Geometry: final body of the model. Coordinates: model frame, mm. Face numbers are marked on the shaded views. A direction names the side the tool comes from. Give positions to 0.01 mm unless a question says otherwise; leave off trailing zeros. Write each loop counter-clockwise with the first axis right and the second up, starting at its lowest first coordinate (ties: lowest second). Pieces come first, ordered by that corner, then holes. Notation, with made-up numbers: M 72.5,85.5 L 83.5,85.5 A15 ccw 83.5,104.5 Z; hole C 74,83.5 d1. An arc over 180 degrees is marked long. One line per question, with ' | ' between items.
Autodesk Inventor part; units mm, degrees
ref_plane "YZ Plane" through (0, 0, 0) normal (1, 0, 0) x (0, 1, 0)
ref_plane "XZ Plane" through (0, 0, 0) normal (0, 1, 0) x (-1, 0, 0)
ref_plane "XY Plane" through (0, 0, 0) normal (0, 0, 1) x (1, 0, 0)
sketch "Sketch1" plane through (0, 0, 0) normal (0, 1, 0) x (-1, 0, 0)
  line L0 (0, 0) -> (25.4, 0)
  line L1 (25.4, 0) -> (25.4, -50.8)
  line L2 (25.4, -50.8) -> (0, -50.8)
  line L3 (0, -50.8) -> (0, 0)
  dimension "d0" = 25.4
  dimension "d1" = 50.8
extrude "Extrusion1" add sketch "Sketch1" along normal blind 15.24
shell "Shell1" thickness 2.54 removed faces 1 at (-8.4667, 15.24, -33.8667)
sketch "Sketch3" plane through (-25.4, 0, 0) normal (0, 0, 1) x (1, 0, 0)
  line L0 (19.05, 4.064) -> (6.35, 4.064)
  line L1 (6.35, 4.064) -> (6.35, 9.144)
  line L2 (6.35, 9.144) -> (19.05, 9.144)
  line L3 (19.05, 9.144) -> (19.05, 4.064)
  point P0 (25.4, 0)
  dimension "d20" = 4.064
  dimension "d21" = 12.7
  dimension "d22" = 5.08
  dimension "d23" = 6.35
extrude "Extrusion3" cut sketch "Sketch3" against normal blind 2.54
chamfer "Chamfer1" distance 3.175 angle 45 2 edges at (-19.05, 9.144, -1.27) (-6.35, 9.144, -1.27)
sketch "Sketch5" plane through (-22.86, 2.54, -2.54) normal (0, 1, 0) x (1, 0, 0)
  line L0 (0, 0) -> (5.08, 0)
  line L1 (5.08, 0) -> (5.08, 45.72)
  line L2 (5.08, 45.72) -> (0, 45.72)
  line L3 (0, 45.72) -> (0, 0)
  line L4 (0, 45.72) -> (20.32, 45.72)
  line L5 (20.32, 0) -> (15.24, 0)
  line L6 (15.24, 0) -> (15.24, 45.72)
  line L7 (15.24, 45.72) -> (20.32, 45.72)
  line L8 (20.32, 45.72) -> (20.32, 0)
  point P0 (22.86, -2.54)
  dimension "d29" = 5.08
  dimension "d30" = 5.08
extrude "Extrusion4" cut sketch "Sketch5" against normal blind 2.54
properties part number "nano_enclosure"
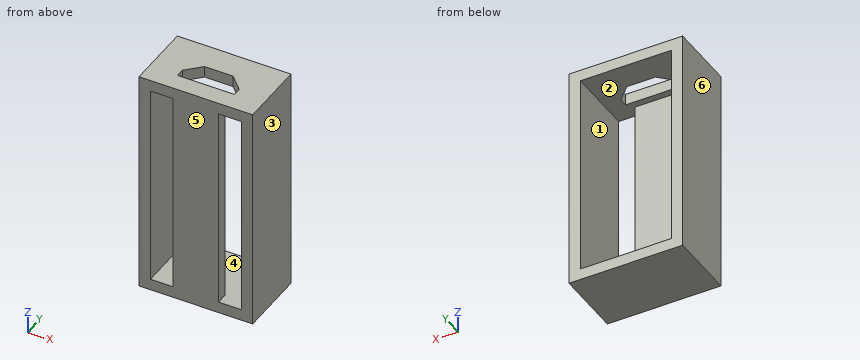
(1) Cut plane A-A, the plane z = -12. Return loops of the section in (x, y).
Working result:
outline: M -25.4,0 L -22.86,0 L -22.86,15.24 L -25.4,15.24 Z; M -17.78,0 L -7.62,0 L -7.62,2.54 L -17.78,2.54 Z; M -2.54,0 L 0,0 L 0,15.24 L -2.54,15.24 Z
(2) First-contact query: P1, Ø1.5, axis at x = -10.5, z = -14.5, coming from the +Y side. Flat tip, straight axial feed; report the tip coordinate or a pass-through.
Working result:
P1: stops at y = 2.54
(3) Set-up query: the marked faces 1, 2 and 3. Return all of +Z, -Z, +X, -X, +Y, -Y with unobstructed straight access to the full face (end or side cutting, diameter ignored); none if empty.
Working result:
face 1: +Y, -Y | face 2: +Y | face 3: +Z, -Z, +X, +Y, -Y
(4) Cut plane B-B, the plane y = 1.75. Return loops of the section in (x, z).
Working result:
outline: M -25.4,-50.8 L 0,-50.8 L 0,0 L -25.4,0 Z; hole M -22.86,-48.26 L -17.78,-48.26 L -17.78,-2.54 L -22.86,-2.54 Z; hole M -7.62,-48.26 L -2.54,-48.26 L -2.54,-2.54 L -7.62,-2.54 Z
(5) Material intervals for L1, parallel to X at y = 1.25, z = -41; L2, parallel to X at y = 10.75, z = -25.5; L3, parallel to Z at x = -17.5, y = 8.75, sorted ascending. Write a range as [from, to].
Working result:
L1: x = [-25.4, -22.86], [-17.78, -7.62], [-2.54, 0] | L2: x = [-25.4, -22.86], [-2.54, 0] | L3: z = [-50.8, -48.26], [-2.54, 0]
(6) Cut plane C-C, the plane x = -3.5. Return loops of the section in (y, z).
Working result:
outline: M 0,-50.8 L 15.24,-50.8 L 15.24,-48.26 L 0,-48.26 Z; M 0,-2.54 L 15.24,-2.54 L 15.24,0 L 0,0 Z
(7) Draft query along X for the marked faces 4, 5 and 6. Return one class per face: released by +X, released by -X, zero draft, split by the parting line, or undercut.
Working result:
face 4: undercut | face 5: zero draft | face 6: released by -X
(8) Cut plane D-D, the plane y = 13.5. Return loops of the section in (x, z).
Working result:
outline: M -25.4,-50.8 L 0,-50.8 L 0,0 L -25.4,0 Z; hole M -22.86,-48.26 L -2.54,-48.26 L -2.54,-2.54 L -22.86,-2.54 Z
